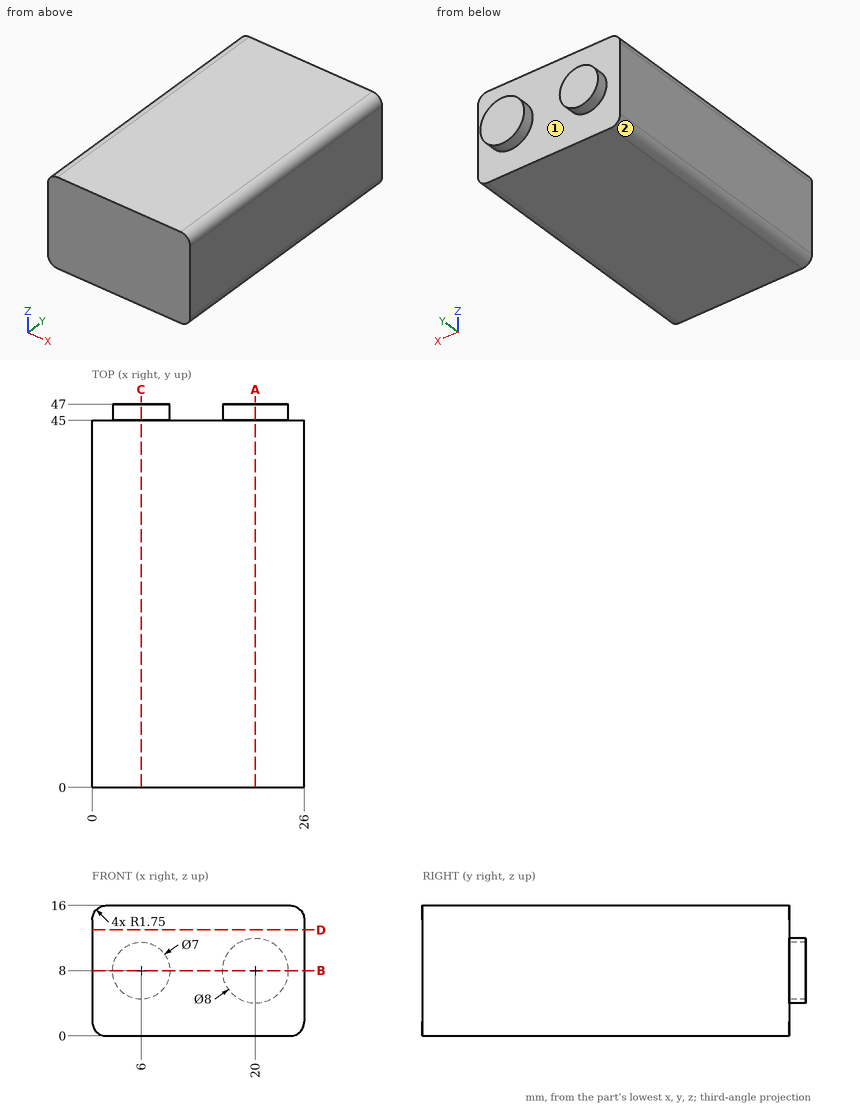
Here's the drawing with two shaded views (mm, measured from the low corner). I have some questions. A direction names the side the tool comes from. Give positions to 0.01 mm unless a question says otherwise; leave off trailing zeros. Order: outer loops, then holes, each group sorted by start corner. A loop starts at its lowest first (then second) coordinate and runs counter-clockwise, first axis right, second up.
Q1. Suppose I cut it at D-D, the plane z = 13. Write out the boundary of the cut face in (x, y).
Q2. Suppose I cut it at A-A, the plane x = 20. Write out the boundary of the cut face in (y, z).
Q3. Suppose I cut it at C-C, the plane x = 6. Write out the boundary of the cut face in (y, z).
Q4. I'm going to push a flat-ended pin straight in: P1, Ø1.5, axis at x = 6, z = 13, coming from the +Y side. Where does the tip first touch, or does it pass through?
Q5. If I drill on line 1 along Y through (x, z) = (3.25, 14); line 2 along Z through (x, y) = (24.75, 10); line 3 along X through (y, z) = (19.5, 1), over which ranges is the centre line in solid material (lowest first)?
Q6. For the marked faces 1 and 2, which set-ups out of +Z, -Z, +X, -X, +Y, -Y let a thin tool reach every point of the face, with its end or its side?
Q7. Suppose I cut it at B-B, the plane z = 8. Write out the boundary of the cut face in (x, y).
Solution:
1. outline: (0, 0) - (26, 0) - (26, 45) - (0, 45) - close
2. outline: (0, 0) - (45, 0) - (45, 4) - (47, 4) - (47, 12) - (45, 12) - (45, 16) - (0, 16) - close
3. outline: (0, 0) - (45, 0) - (45, 4.5) - (47, 4.5) - (47, 11.5) - (45, 11.5) - (45, 16) - (0, 16) - close
4. P1: stops at y = 45
5. line 1: y = 0 to 45
5. line 2: z = 0.07 to 15.93
5. line 3: x = 0.17 to 25.83
6. face 1: +Y
6. face 2: -Z, -X, +Y, -Y
7. outline: (0, 0) - (26, 0) - (26, 45) - (24, 45) - (24, 47) - (16, 47) - (16, 45) - (9.5, 45) - (9.5, 47) - (2.5, 47) - (2.5, 45) - (0, 45) - close
